```python
from build123d import *

# Parameters (mm, degrees)
F0_W      = 25.4
F0_H      = 25.4
F1_DEPTH  = 25.4
F2_R      = 6.3119
F3_DEPTH  = 8.0264
F7_W      = 25.4
F7_H      = 12.7
F8_DEPTH  = 50.8
F9_DEPTH  = 25.4
F11_DEPTH = 50.8
F12_DEPTH = 50.8
F13_DEPTH = 25.4
F14_DEPTH = 50.8
F15_DEPTH = 50.8


with BuildPart() as f1:
    # F0 (on Front) → F1 (new body)
    with BuildSketch(Plane.XZ):
        with Locations((-12.7, 12.7)):
            Rectangle(F0_W, F0_H)
    extrude(amount=F1_DEPTH)

    # F2 (on Top) → F3 (cut)
    with BuildSketch(Plane.XY):
        Polygon((-7.2579364777, -22.1902352696), (-1.7601834075, -12.7321523755), (-7.2022469298, -3.2419171059), (-18.1420635223, -3.2097647304), (-23.6398165925, -12.6678476245), (-18.1977530702, -22.1580828941), align=None)
        with Locations((-12.7, -12.7)):
            Circle(F2_R, mode=Mode.SUBTRACT)
    extrude(amount=F3_DEPTH, mode=Mode.SUBTRACT)

    # F5 (on offset) → F6 (revolve)
    with BuildSketch(Plane.XZ.offset(12.7)):
        with BuildLine():
            Line((-12.7, 25.4), (-12.7, 38.1))
            ThreePointArc((-12.7, 38.1), (-21.6802561211, 34.3802561211), (-25.4, 25.4))
            Line((-25.4, 25.4), (-12.7, 25.4))
        make_face()
    revolve(axis=Axis((-12.7, -12.7, 31.75), (0, 0, 1)))

    # F7 (on Right) → F8 (join)
    with BuildSketch(Plane.YZ):
        with Locations((-12.7, 26.67)):
            Rectangle(F7_W, F7_H)
    extrude(amount=-F8_DEPTH)

    # F7 (on Right) → F9 (join)
    with BuildSketch(Plane.YZ):
        with Locations((-12.7, 26.67)):
            Rectangle(F7_W, F7_H)
    extrude(amount=F9_DEPTH)

    # F10 (on face) → F11 (cut)
    with BuildSketch(Plane.XY.offset(33.02)):
        with BuildLine():
            add(Edge.make_bspline(
                [(-12.7, 0), (-17.3658879301, -0.2554953412), (-25.0834624368, -0.8683027323), (-31.191647473, -2.7804494515), (-34.6991875165, -5.0056243623), (-36.660656333, -6.4021432772), (-38.1, -7.8327860683)],
                knots=[0, 0, 0, 0, 0.3525244295, 0.5971540178, 0.7887122331, 1, 1, 1, 1], degree=3))
            Line((-12.7, 0), (-38.1, 0))
            Line((-38.1, 0), (-38.1, -7.8327860683))
        make_face()
    extrude(amount=-F11_DEPTH, mode=Mode.SUBTRACT)

    # F10 (on face) → F12 (cut)
    with BuildSketch(Plane.XY.offset(33.02)):
        with BuildLine():
            add(Edge.make_bspline(
                [(-12.7, -25.4), (-17.3987553045, -24.9769857908), (-25.3139427174, -24.6420420616), (-30.0058965126, -22.5738416728), (-34.8725168747, -19.6257840333), (-36.0709987581, -18.2458739728), (-38.1, -16.4399109781)],
                knots=[0, 0, 0, 0, 0.3473379926, 0.5672748801, 0.7821069123, 1, 1, 1, 1], degree=3))
            Line((-38.1, -16.4399109781), (-38.1, -25.4))
            Line((-38.1, -25.4), (-12.7, -25.4))
        make_face()
    extrude(amount=-F12_DEPTH, mode=Mode.SUBTRACT)

    # F10 (on face) → F13 (cut)
    with BuildSketch(Plane.XY.offset(33.02)):
        with BuildLine():
            Line((-38.1, -7.8327860683), (-38.1, 0))
            Line((-38.1, 0), (-50.8, 0))
            Line((-50.8, 0), (-50.8, -25.4))
            Line((-50.8, -25.4), (-38.1, -25.4))
            Line((-38.1, -25.4), (-38.1, -16.4399109781))
            ThreePointArc((-38.1, -16.4399109781), (-49.1192451421, -12.1363485232), (-38.1, -7.8327860683))
        make_face()
    extrude(amount=-F13_DEPTH, mode=Mode.SUBTRACT)

    # F10 (on face) → F14 (cut)
    with BuildSketch(Plane.XY.offset(33.02)):
        with BuildLine():
            Line((25.4, 0), (-12.7, 0))
            add(Edge.make_bspline(
                [(-12.7, 0), (-8.0341120699, -0.2554953412), (-0.3165375632, -0.8683027323), (5.791647473, -2.7804494515), (9.2991875165, -5.0056243623), (11.260656333, -6.4021432772), (12.7, -7.8327860683)],
                knots=[0, 0, 0, 0, 0.3525244295, 0.5971540178, 0.7887122331, 1, 1, 1, 1], degree=3))
            ThreePointArc((12.7, -7.8327860683), (19.6793093563, -6.22144334), (23.7192451421, -12.1363485232))
            ThreePointArc((23.7192451421, -12.1363485232), (19.6793093563, -18.0512537064), (12.7, -16.4399109781))
            add(Edge.make_bspline(
                [(-12.7, -25.4), (-8.0012446955, -24.9769857908), (-0.0860572826, -24.6420420616), (4.6058965126, -22.5738416728), (9.4725168747, -19.6257840333), (10.6709987581, -18.2458739728), (12.7, -16.4399109781)],
                knots=[0, 0, 0, 0, 0.3473379926, 0.5672748801, 0.7821069123, 1, 1, 1, 1], degree=3))
            Line((-12.7, -25.4), (25.4, -25.4))
            Line((25.4, -25.4), (25.4, 0))
        make_face()
    extrude(amount=-F14_DEPTH, mode=Mode.SUBTRACT)

    # F2 (on Top) → F15 (cut)
    with BuildSketch(Plane.XY):
        with Locations((-12.7, -12.7)):
            Circle(F2_R)
    extrude(amount=F15_DEPTH, mode=Mode.SUBTRACT)


solid = f1.part
```
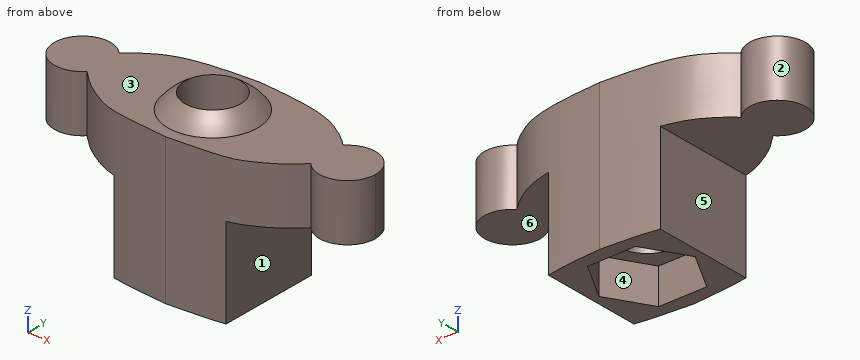
Source: CAD feature listing. Evaluate the final solid. Frame: model axes, mm. Face numbers are marked on the shaded views. A direction names the side the tool comes from. Round coordinates to 2 decimals unless told otherwise and drop trailing zeros. Loops run counter-clockwise (first coordinate to the right, second up) from the corner with the lowest first, then second, coordinate; pieces in that order, holes last. Notation, with made-up numbers: M -38.5,-39 L -17.5,-39 A12 ccw -17.5,-21 Z; hole C 4,-39 d3. An arc over 180 degrees is marked long. Use a Markdown table: item, result. Add a question column.
1. Section query A-A on x = 18. Return the cut outline in (y, z).
2. Mould query, pull axis X, two halves, no side actions, for the marked faces 1, 2 and 3. Classes: pulls with the +X half, pulls with the -X half, needs draft (parallel to the pull), parting line crosses it, or undercut.
3. Line query: line 1 (Y direction, x = -12.7, z = 14.5); line 2 (X direction, y = -6, z = 17). Output: solid intervals per line, ascending.
4. Contact query for flat-ended pins moving along their axis: P1, Ø2, axis at x = -8, z = 13.5, coming from the -Y side; P2, Ø6, axis at y = -7.5, z = 5.5, coming from the +X side; P3, Ø7.5, axis at x = -12.7, y = -12.7, coming from the -Z side; P4, Ø12, axis at x = -28.5, z = 24.5, coming from the -Y side. Output: stop coordinate, or through.
5. Section query B-B on x = -40.5. Return the cut outline in (y, z), then the cut area to 3 significant figures.
6. Reachability of the marked faces 4, 5 and 6 from +Z, -Z, +X, -X, +Y, -Y: full face, straight path, thin tool, end or side. Return the list, or none.
Reported:
| question | item | result |
|---|---|---|
| 1 | outline | M -18.45,20.32 L -5.82,20.32 L -5.82,33.02 L -18.45,33.02 Z |
| 2 | face 1 | pulls with the +X half |
| 2 | face 2 | undercut |
| 2 | face 3 | needs draft |
| 3 | line 1 | y = -25.4 to -19.01, -6.39 to 0 |
| 3 | line 2 | x = -25.4 to 0 |
| 4 | P1 | stops at y = -25.1 |
| 4 | P2 | stops at x = 0 |
| 4 | P3 | passes through |
| 4 | P4 | stops at y = -24.57 |
| 5 | outline | M -18.07,20.32 L -6.21,20.32 L -6.21,33.02 L -18.07,33.02 Z |
| 5 | area | 151 mm² |
| 6 | face 4 | -Z |
| 6 | face 5 | -Z, -X, +Y, -Y |
| 6 | face 6 | -Z, +X, +Y, -Y |
